Here's how the part is built. I have some questions about the finished solid (model axes, mm). A direction names the side the tool comes from. Round coordinates to 2 decimals unless told otherwise and drop trailing zeros. Loops run counter-clockwise (first coordinate to the right, second up) from the corner with the lowest first, then second, coordinate; pieces in that order, holes last. Notation, with made-up numbers: (30.25, 22.25) -> (61.25, 22.25) arc R17 cw to (61.25, 44.25) -> close; hole circle Ø1 at (-32.75, -14.75). An arc over 180 degrees is marked (long way). One line per item, written item: value. Start each with the question number.
```python
from build123d import *

# Parameters (mm, degrees)
CYLINDER002_R       = 2
CYLINDER002_DEPTH   = 10
SKETCH007_W         = 17
SKETCH007_H         = 8
PAD002_DEPTH        = 18
HOLE003_D           = 3
HOLE003_DEPTH       = 10
HOLE003_CSINK_D     = 6.1
HOLE003_CSINK_ANGLE = 90
HOLE003_TIPS_R      = 1.5
SKETCH009_R         = 3
HOLE004_DEPTH       = 7


with BuildPart() as cylinder002:
    # Cylinder002 → Cylinder002 (new body)
    with BuildSketch(Plane(origin=(-5.5, -9, 2.8), x_dir=(1, 0, 0), z_dir=(0, -1, 0))):
        Circle(CYLINDER002_R)
    extrude(amount=CYLINDER002_DEPTH)


with BuildPart() as cut002004:
    # Sketch007 → Pad002 (new body)
    with BuildSketch(Plane.XZ):
        Rectangle(SKETCH007_W, SKETCH007_H)
    extrude(amount=PAD002_DEPTH)

    # Hole003
    with Locations(Plane.XZ.offset(18)):
        with Locations((0, 0)):
            CounterSinkHole(HOLE003_D / 2, HOLE003_CSINK_D / 2, depth=HOLE003_DEPTH, counter_sink_angle=HOLE003_CSINK_ANGLE)

    # Hole003 tips → Hole003 tip 1 section 0
    with BuildSketch(Plane.XZ.offset(8), mode=Mode.PRIVATE) as hole003_tip_1_s0:
        Circle(HOLE003_TIPS_R)
    loft([hole003_tip_1_s0.sketch, Vertex(0, -7.098709, 0)], mode=Mode.SUBTRACT)

    # Sketch009 (on Face1 of Hole003) → Hole004 (cut)
    with BuildSketch(Plane(origin=(0, 0, 4), x_dir=(-1, 0, 0), z_dir=(0, 0, 1))):
        with Locations((0, 6)):
            Circle(SKETCH009_R)
    extrude(amount=-HOLE004_DEPTH, mode=Mode.SUBTRACT)

    # Cut002004: cut Cylinder002
    add(cylinder002.part, mode=Mode.SUBTRACT)


solid = cut002004.part
```
Q1. I want a section at C-C on x = 0. Please give me the cut outline in (y, z), plus the area to 3 significant figures.
Q2. I want a section at B-B on z = 0. Please give me the cut outline in (x, y), plus the area to 3 significant figures.
Q3. Will these pins go through, and if not, where does the flat tip stop? P1, Ø1.5, axis at x = 5, z = -2.5, coming from the +Y side; P2, Ø1, axis at x = -6, z = 3, coming from the -Y side; P3, Ø1.5, axis at x = 0.5, z = -2, coming from the -Y side.
Q4. If we mould it in two halves opening along X, with no side actions, what happens to faces 1 (the flat face through (8.5, -9, 0)), 2 (the cylindrical face through (-1.386, -12.469, -0.575)), 3 (the flat face through (2, -18, -3))? For each: released by +X, released by -X, zero draft, split by the parting line, or undercut.
Q5. I want a section at D-D on y = -6. Please give me the cut outline in (x, z), plus the area to 3 significant figures.
Q6. If I drill on line 1 along X through (y, z) = (-6, -1); line 2 along X through (y, z) = (-10.5, 0); line 3 along Y through (x, z) = (-1, -2), over which ranges is the centre line in solid material (lowest first)?
Q7. I want a section at A-A on y = -15.25. Please give me the cut outline in (x, z).
Q8. Which directions (+Z, -Z, +X, -X, +Y, -Y) give clear straight access to the entire face, cutting with the end or side of a thin tool? Please do faces 4 (the cylindrical face through (-5.56, -13.44, 0.8)), 5 (the flat face through (0, 0, 0)), 6 (the flat face through (0, -6, -3)), 7 (the flat face through (2, -9, 4)).
Answers below:
1. outline: (-18, -4) -> (0, -4) -> (0, 4) -> (-3, 4) -> (-3, -3) -> (-9, -3) -> (-9, -1.5) -> (-16.45, -1.5) -> (-18, -3.05) -> close; (-18, 3.05) -> (-16.45, 1.5) -> (-9, 1.5) -> (-9, 4) -> (-18, 4) -> close
1. area: 72.6 mm^2
2. outline: (-8.5, -18) -> (-3.05, -18) -> (-1.5, -16.45) -> (-1.5, -8.6) arc R3 cw (long way) to (1.5, -8.6) -> (1.5, -16.45) -> (3.05, -18) -> (8.5, -18) -> (8.5, 0) -> (-8.5, 0) -> close
2. area: 248 mm^2
3. P1: stops at y = 0
3. P2: stops at y = -9
3. P3: stops at y = -17.76
4. face 1: released by +X
4. face 2: undercut
4. face 3: zero draft
5. outline: (-8.5, -4) -> (8.5, -4) -> (8.5, 4) -> (3, 4) -> (3, -3) -> (-3, -3) -> (-3, 4) -> (-8.5, 4) -> close
5. area: 94.0 mm^2
6. line 1: x = -8.5 to -3, 3 to 8.5
6. line 2: x = -8.5 to -1.5, 1.5 to 8.5
6. line 3: y = -17.19 to -8.83, -3.17 to 0
7. outline: (-8.5, -4) -> (8.5, -4) -> (8.5, 4) -> (-3.9, 4) arc R2 cw (long way) to (-7.1, 4) -> (-8.5, 4) -> close; hole circle Ø3 at (0, 0)
8. face 4: -Y
8. face 5: +Z, -Z, +X, -X, +Y
8. face 6: +Z
8. face 7: +Z, +X, -X, +Y, -Y
